Read the model definition and answer for the solid it produces. Units are mm, in the model's axes. A direction names the side the tool comes from. Coordinates: 2 decimals unless noted, no trailing zeros. Order: outer loops, then holes, each group sorted by start corner. A loop starts at its lowest first (then second) coordinate and runs counter-clockwise, first axis right, second up. Notation, with made-up numbers: M 26,-34.5 L 83,-34.5 A5 cw 83,-29.5 Z; hole C 66.25,7 d1. An arc over 180 degrees is marked long. Use a Markdown table: item, result. Add a question column.
1) For faces 4 (the face through (1, 28, 28)), 5 (the face through (35, 0, 33)), 6 (the face through (69, 28, 28)), 7 (the face through (35, 5, 35)), 8 (the face through (16.42, 2.54, 20.12)), determine the directions among +Z, -Z, +X, -X, +Y, -Y from which every point of the face is accessible in a straight line to the end or side of a thin tool.
2) Find the intervals of material crossed by probe 1 along X at (y, z) = (27.6, 25); probe 2 along Z at (x, y) = (35, 1.3); probe 3 along Y at (x, z) = (24, 44.5), in increasing order. Write a range as [from, to].
3) Find section A-A on z = 17.5. Write down the section's boundary in (x, y).
4) Find section D-D on z = 40. Write down the section's boundary in (x, y).
5) The mould has two halves that part along X. Classify faces 1 (the face through (51.01, 26.87, 23.86)), 2 (the face through (35, 15, 0)), 3 (the face through (0, 4, 21)): released by +X, released by -X, zero draft, split by the parting line, or undercut.
6) Find section C-C on y = 6.5. Write down the section's boundary in (x, z), plus the area to 3 significant figures.
7) Each of these flat-tipped pins is pushed along its axis until it touches: pin 1 Ø4 at (x, y) = (36, 28.5) entering from +Z; pin 2 Ø2 at (x, z) = (48, 36) entering from +Y; pin 3 Ø8 at (x, y) = (19, 12.5) entering from +Z. Where does it stop, or does it pass through?
8) Find section B-B on x = 17.5. Write down the section's boundary in (y, z).
from build123d import *

# Parameters (mm, degrees)
CYLINDER001_R         = 1.8
CYLINDER001_DEPTH     = 5
CYLINDER_R            = 5
CYLINDER_DEPTH        = 30
ARRAY_X_COUNT         = 3
ARRAY_X_PITCH         = 17.5
ARRAY_PLACEMENT_ANGLE = 90
BOX001_W              = 70
BOX001_H              = 20
BOX001_DEPTH          = 50
BOX002_W              = 70
BOX002_H              = 15
BOX002_DEPTH          = 30
FILLET002_R           = 5
BOX_W                 = 70
BOX_H                 = 15
BOX_DEPTH             = 55
FILLET001_R           = 5
CHAMFER_SIZE          = 9.1


with BuildPart() as screw_hole:
    # Cylinder001 → Cylinder001 (new body)
    with BuildSketch(Plane.XY):
        Circle(CYLINDER001_R)
    extrude(amount=CYLINDER001_DEPTH)


with BuildPart() as screw_driver_hole:
    # Cylinder → Cylinder (new body)
    with BuildSketch(Plane.XY.offset(7)):
        Circle(CYLINDER_R)
    extrude(amount=CYLINDER_DEPTH)


with BuildPart() as hole_array:
    # Cone → Cone (revolve)
    with BuildSketch(Plane(origin=(0, 0, 5), x_dir=(1, 0, 0), z_dir=(0, -1, 0))):
        Polygon((0, 0), (1.8, 0), (3, 2), (0, 2), align=None)
    revolve(axis=Axis((0, 0, 5), (0, 0, 1)))

    # Fusion: union screw hole, screw driver hole
    add(screw_hole.part)
    add(screw_driver_hole.part)

    # Array X: hole array ×3


with BuildPart() as hole_array_1:
    add(hole_array.part)
    with Locations(*[(i * ARRAY_X_PITCH, 0, 0) for i in range(1, ARRAY_X_COUNT)]):
        add(hole_array.part)


with BuildPart() as hole_array_2:
    # Array placement: moved
    add(hole_array_1.part.moved(Location((17.5, 32, 25))).rotate(Axis((17.5, 32, 25), (1, 0, 0)), ARRAY_PLACEMENT_ANGLE))


with BuildPart() as internal_cube:
    # Box001 → Box001 (new body)
    with BuildSketch(Plane(origin=(0, 5, 6), x_dir=(1, 0, 0), z_dir=(0, 0, 1))):
        with Locations((35, 10)):
            Rectangle(BOX001_W, BOX001_H)
    extrude(amount=BOX001_DEPTH)


with BuildPart() as external_hole_side_half_fillet:
    # Box002 → Box002 (new body)
    with BuildSketch(Plane(origin=(0, 15, 0), x_dir=(1, 0, 0), z_dir=(0, 0, 1))):
        with Locations((35, 7.5)):
            Rectangle(BOX002_W, BOX002_H)
    extrude(amount=BOX002_DEPTH)

    # Fillet002
    fillet002_edges = [external_hole_side_half_fillet.edges().sort_by_distance(p)[0] for p in [
        (0, 22.5, 30),
        (0, 22.5, 0),
        (70, 22.5, 30),
        (70, 22.5, 0),
    ]]
    fillet(fillet002_edges, radius=FILLET002_R)


with BuildPart() as wire_hanger_cut001:
    # Box → Box (new body)
    with BuildSketch(Plane.XY):
        with Locations((35, 7.5)):
            Rectangle(BOX_W, BOX_H)
    extrude(amount=BOX_DEPTH)

    # Fillet001
    fillet001_edges = [wire_hanger_cut001.edges().sort_by_distance(p)[0] for p in [
        (0, 7.5, 55),
        (0, 7.5, 0),
        (70, 7.5, 55),
        (70, 7.5, 0),
    ]]
    fillet(fillet001_edges, radius=FILLET001_R)

    # Fusion001: union external hole side half fillet
    add(external_hole_side_half_fillet.part)

    # Cut: cut internal cube
    add(internal_cube.part, mode=Mode.SUBTRACT)

    # Chamfer
    chamfer_edges = [wire_hanger_cut001.edges().sort_by_distance(p)[0] for p in [
        (35, 5, 6),
        (35, 25, 6),
    ]]
    chamfer(chamfer_edges, length=CHAMFER_SIZE)

    # Cut001: cut hole array
    add(hole_array_2.part, mode=Mode.SUBTRACT)


solid = wire_hanger_cut001.part
Check result:
| question | item | result |
|---|---|---|
| 1 | face 4 | +Z, -X, +Y |
| 1 | face 5 | +Z, -Z, +X, -X, -Y |
| 1 | face 6 | +Z, +X, +Y |
| 1 | face 7 | +Z, +X, -X |
| 1 | face 8 | -Y |
| 2 | probe 1 | x = [0, 15.7], [19.3, 33.2], [36.8, 50.7], [54.3, 70] |
| 2 | probe 2 | z = [0, 20], [30, 55] |
| 2 | probe 3 | y = [0, 5] |
| 3 | outline | M 0,0 L 70,0 L 70,5 L 0,5 Z; M 0,25 L 70,25 L 70,30 L 0,30 Z |
| 4 | outline | M 0,0 L 70,0 L 70,5 L 0,5 Z |
| 5 | face 1 | undercut |
| 5 | face 2 | zero draft |
| 5 | face 3 | released by -X |
| 6 | outline | M 0,5 A5 ccw 5,0 L 65,0 A5 ccw 70,5 L 70,13.6 L 0,13.6 Z |
| 6 | area | 941 mm2 |
| 7 | pin 1 | stops at z = 30 |
| 7 | pin 2 | stops at y = 5 |
| 7 | pin 3 | stops at z = 11.6 |
| 8 | outline | M 0,0 L 30,0 L 30,23.2 L 27,23.2 L 25,22 L 25,15.1 L 15.9,6 L 14.1,6 L 5,15.1 L 5,20 L 0,20 Z; M 0,30 L 5,30 L 5,55 L 0,55 Z; M 25,28 L 27,26.8 L 30,26.8 L 30,30 L 25,30 Z |
